```python
from build123d import *

# Parameters (mm, degrees)
SCHIZZO1_W                        = 94.2
SCHIZZO1_H                        = 61
ESTRUSIONE_ESTRUSIONE1_DEPTH      = 4
SCHIZZO2_W                        = 108
SCHIZZO2_H                        = 61.6
ESTRUSIONE_ESTRUSIONE2_DEPTH      = 1.6
ESTRUSIONE_ESTRUSIONE3_DEPTH      = 1.3
ESTRUSIONE_ESTRUSIONE3_DEPTH_BACK = 9.9
SCHIZZO4_W                        = 2.5
SCHIZZO4_H                        = 35.8
SCHIZZO6_R                        = 1.5
TAGLIO_ESTRUSIONE1_DEPTH          = 2
SCHIZZO7_W                        = 27
SCHIZZO7_H                        = 17
ESTRUSIONE_ESTRUSIONE4_DEPTH      = 3


with BuildPart() as part:
    # Schizzo1 → Estrusione-Estrusione1 (new body)
    with BuildSketch(Plane(origin=(0, 0, 0), x_dir=(1, 0, 0), z_dir=(0, 1, 0))):
        with Locations((47.1, 30.5)):
            Rectangle(SCHIZZO1_W, SCHIZZO1_H)
    extrude(amount=ESTRUSIONE_ESTRUSIONE1_DEPTH)

    # Schizzo2 → Estrusione-Estrusione2 (add)
    with BuildSketch(Plane.XZ):
        with Locations((47, -30.5)):
            Rectangle(SCHIZZO2_W, SCHIZZO2_H)
    extrude(amount=ESTRUSIONE_ESTRUSIONE2_DEPTH)

    # Schizzo4 → Estrusione-Estrusione3 (add, two sides: drawn at the far end of the back side and taken through both)
    with BuildSketch(Plane(origin=(0, 0, 0), x_dir=(1, 0, 0), z_dir=(0, 1, 0)).offset(-ESTRUSIONE_ESTRUSIONE3_DEPTH_BACK)):
        with Locations((98.95, 30.4)):
            Rectangle(SCHIZZO4_W, SCHIZZO4_H)
    extrude(amount=ESTRUSIONE_ESTRUSIONE3_DEPTH + ESTRUSIONE_ESTRUSIONE3_DEPTH_BACK)

    # Schizzo6 → Taglio-Estrusione1 (cut)
    with BuildSketch(Plane(origin=(0, 0, 0), x_dir=(1, 0, 0), z_dir=(0, 1, 0))):
        with Locations(Location((-4, 57.8, 0), (0, 0, 270))):
            Circle(SCHIZZO6_R)
        with Locations(Location((-4, 3.2, 0), (0, 0, 270))):
            Circle(SCHIZZO6_R)
        with Locations(Location((98, 57.8, 0), (0, 0, 270))):
            Circle(SCHIZZO6_R)
        with Locations(Location((98, 3.2, 0), (0, 0, 270))):
            Circle(SCHIZZO6_R)
    extrude(amount=-TAGLIO_ESTRUSIONE1_DEPTH, mode=Mode.SUBTRACT)

    # Schizzo7 → Estrusione-Estrusione4 (add)
    with BuildSketch(Plane.XZ.offset(1.6)):
        with Locations((34.5, -12.7)):
            Rectangle(SCHIZZO7_W, SCHIZZO7_H)
    extrude(amount=ESTRUSIONE_ESTRUSIONE4_DEPTH)


solid = part.part
```
Could you check a few things on this model? Use its own coordinates, in mm. A direction names the side the tool comes from. Give positions to 0.01 mm unless a question says otherwise; leave off trailing zeros. Loops run counter-clockwise (first coordinate to the right, second up) from the corner with the lowest first, then second, coordinate; pieces in that order, holes last. Notation, with made-up numbers: (1, -21.5) -> (30, -21.5) arc R15 ccw to (30, 1.5) -> close; hole circle Ø10 at (-9.5, 12). An arc over 180 degrees is marked (long way). Put each result on its own line as item: value.
(1) Thinking about a two-plate mould opening in Z: for faces 4 (the face through (46, 2, -61)), 5 (the face through (46, 4, -31)), 6 (the face through (-4.9, -0.8, -59)), which applies, pulls with the +Z half, pulls with the -Z half, needs draft (parallel to the pull), parting line crosses it, or undercut?
Computed:
face 4: pulls with the -Z half
face 5: needs draft
face 6: undercut
(2) Imagine slicing it at D-D on x = 74. Write out the boundary of the cut face in (y, z).
Computed:
outline: (-1.6, -61.3) -> (0, -61.3) -> (0, -61) -> (4, -61) -> (4, 0) -> (0, 0) -> (0, 0.3) -> (-1.6, 0.3) -> close
(3) Imagine slicing it at A-A on z = -57.8. Write out the boundary of the cut face in (x, y).
Computed:
outline: (-7, -1.6) -> (-5.5, -1.6) -> (-5.5, 0) -> (-7, 0) -> close; (-2.5, -1.6) -> (96.5, -1.6) -> (96.5, 0) -> (94.2, 0) -> (94.2, 4) -> (0, 4) -> (0, 0) -> (-2.5, 0) -> close; (99.5, -1.6) -> (101, -1.6) -> (101, 0) -> (99.5, 0) -> close
(4) Please list where these lines run through material, in increasing order: probe 1 along Z at (x, y) = (98, -1.05); probe 2 along X at (y, z) = (1.25, -19); probe 3 along X at (y, z) = (-0.8, -57.8). Write a range as [from, to].
Computed:
probe 1: [-61.3, -59.3], [-56.3, -4.7], [-1.7, 0.3]
probe 2: [0, 94.2], [97.7, 100.2]
probe 3: [-7, -5.5], [-2.5, 96.5], [99.5, 101]
(5) Imagine slicing it at C-C on z = -44. Write out the boundary of the cut face in (x, y).
Computed:
outline: (-7, -1.6) -> (97.7, -1.6) -> (97.7, -9.9) -> (100.2, -9.9) -> (100.2, -1.6) -> (101, -1.6) -> (101, 0) -> (100.2, 0) -> (100.2, 1.3) -> (97.7, 1.3) -> (97.7, 0) -> (94.2, 0) -> (94.2, 4) -> (0, 4) -> (0, 0) -> (-7, 0) -> close
(6) For faces 1 (the face through (46, 2, 0)), 2 (the face through (21, -3, -13)), 3 (the face through (34, -3, -21.2)), which set-ups out of +Z, -Z, +X, -X, +Y, -Y let a thin tool reach every point of the face, with its end or its side?
Computed:
face 1: +Z, +X, -X, +Y
face 2: +Z, -Z, -X, -Y
face 3: -Z, -X, -Y
(7) Imagine slicing it at B-B on x = -4. Write out the boundary of the cut face in (y, z).
Computed:
outline: (-1.6, -61.3) -> (0, -61.3) -> (0, -59.3) -> (-1.6, -59.3) -> close; (-1.6, -56.3) -> (0, -56.3) -> (0, -4.7) -> (-1.6, -4.7) -> close; (-1.6, -1.7) -> (0, -1.7) -> (0, 0.3) -> (-1.6, 0.3) -> close
(8) I'm going to push flat-ended pins straight in: pin 1 Ø2 at (y, z) = (2.5, -27.5) entering from +X; pin 2 Ø0.7 at (x, y) = (99, 0.5) entering from +Z; pin 3 Ø1.5 at (x, z) = (34.5, -31) entering from -Y. Where does each tip first touch, or does it pass through?
Computed:
pin 1: x = 94.2
pin 2: z = -12.5
pin 3: y = -1.6
